from build123d import *

# Parameters (mm, degrees)
CYLINDER904_R               = 1.5
CYLINDER904_DEPTH           = 20
CYLINDER904_PLACEMENT_ANGLE = 45
CYLINDER907_R               = 1.5
CYLINDER907_DEPTH           = 20
CYLINDER902_R               = 1.5
CYLINDER902_DEPTH           = 20
CYLINDER902_PLACEMENT_ANGLE = 135
CYLINDER901_R               = 1.5
CYLINDER901_DEPTH           = 20
CYLINDER903_R               = 1.5
CYLINDER903_DEPTH           = 20
CYLINDER903_PLACEMENT_ANGLE = 225
CYLINDER905_R               = 1.5
CYLINDER905_DEPTH           = 20
CYLINDER906_R               = 1.5
CYLINDER906_DEPTH           = 20
CYLINDER906_PLACEMENT_ANGLE = 45
CYLINDER898_R               = 1.5
CYLINDER898_DEPTH           = 20
COMPOUND256_PLACEMENT_ANGLE = 22.5
BOX408_W                    = 6
BOX408_H                    = 8
BOX408_DEPTH                = 2
BOX408_PLACEMENT_ANGLE      = 45
BOX404_W                    = 6
BOX404_H                    = 8
BOX404_DEPTH                = 2
BOX415_W                    = 6
BOX415_H                    = 8
BOX415_DEPTH                = 2
BOX415_PLACEMENT_ANGLE      = 135
BOX407_W                    = 6
BOX407_H                    = 8
BOX407_DEPTH                = 2
BOX412_W                    = 6
BOX412_H                    = 8
BOX412_DEPTH                = 2
BOX412_PLACEMENT_ANGLE      = 225
BOX128_W                    = 6
BOX128_H                    = 8
BOX128_DEPTH                = 2
BOX414_W                    = 6
BOX414_H                    = 8
BOX414_DEPTH                = 2
BOX414_PLACEMENT_ANGLE      = 45
BOX413_W                    = 6
BOX413_H                    = 8
BOX413_DEPTH                = 2
COMPOUND780_PLACEMENT_ANGLE = 22.5
CYLINDER888_R               = 1.5
CYLINDER888_DEPTH           = 20
CYLINDER897_R               = 1.5
CYLINDER897_DEPTH           = 20
CYLINDER896_R               = 1.5
CYLINDER896_DEPTH           = 20
CYLINDER900_R               = 1.5
CYLINDER900_DEPTH           = 20
BOX409_W                    = 6
BOX409_H                    = 2
BOX409_DEPTH                = 6
BOX406_W                    = 6
BOX406_H                    = 2
BOX406_DEPTH                = 6
BOX411_W                    = 6
BOX411_H                    = 2
BOX411_DEPTH                = 6
BOX410_W                    = 6
BOX410_H                    = 2
BOX410_DEPTH                = 6
TUBE087_R                   = 52
TUBE087_R_2                 = 42
TUBE087_DEPTH               = 8


with BuildPart() as obj1:
    # Cylinder904 → Cylinder904 (new body)
    with BuildSketch(Plane.XY):
        Circle(CYLINDER904_R)
    extrude(amount=CYLINDER904_DEPTH)


with BuildPart() as obj1_1:
    # Cylinder904 placement: moved
    add(obj1.part.moved(Location((-31.819805, 31.819805, -18))).rotate(Axis((-31.819805, 31.819805, -18), (0, 0, 1)), CYLINDER904_PLACEMENT_ANGLE))


with BuildPart() as obj2:
    # Cylinder907 → Cylinder907 (new body)
    with BuildSketch(Plane(origin=(-45, 0, -18), x_dir=(0, 1, 0), z_dir=(0, 0, 1))):
        Circle(CYLINDER907_R)
    extrude(amount=CYLINDER907_DEPTH)


with BuildPart() as obj3:
    # Cylinder902 → Cylinder902 (new body)
    with BuildSketch(Plane.XY):
        Circle(CYLINDER902_R)
    extrude(amount=CYLINDER902_DEPTH)


with BuildPart() as obj3_1:
    # Cylinder902 placement: moved
    add(obj3.part.moved(Location((-31.819805, -31.819805, -18))).rotate(Axis((-31.819805, -31.819805, -18), (0, 0, 1)), CYLINDER902_PLACEMENT_ANGLE))


with BuildPart() as obj4:
    # Cylinder901 → Cylinder901 (new body)
    with BuildSketch(Plane(origin=(0, -45, -18), x_dir=(-1, 0, 0), z_dir=(0, 0, 1))):
        Circle(CYLINDER901_R)
    extrude(amount=CYLINDER901_DEPTH)


with BuildPart() as obj5:
    # Cylinder903 → Cylinder903 (new body)
    with BuildSketch(Plane.XY):
        Circle(CYLINDER903_R)
    extrude(amount=CYLINDER903_DEPTH)


with BuildPart() as obj5_1:
    # Cylinder903 placement: moved
    add(obj5.part.moved(Location((31.819805, -31.819805, -18))).rotate(Axis((31.819805, -31.819805, -18), (0, 0, 1)), CYLINDER903_PLACEMENT_ANGLE))


with BuildPart() as obj6:
    # Cylinder905 → Cylinder905 (new body)
    with BuildSketch(Plane(origin=(45, 0, -18), x_dir=(0, -1, 0), z_dir=(0, 0, 1))):
        Circle(CYLINDER905_R)
    extrude(amount=CYLINDER905_DEPTH)


with BuildPart() as obj7:
    # Cylinder906 → Cylinder906 (new body)
    with BuildSketch(Plane.XY):
        Circle(CYLINDER906_R)
    extrude(amount=CYLINDER906_DEPTH)


with BuildPart() as obj7_1:
    # Cylinder906 placement: moved
    add(obj7.part.moved(Location((31.819805, 31.819805, -18))).rotate(Axis((31.819805, 31.819805, -18), (0, 0, -1)), CYLINDER906_PLACEMENT_ANGLE))


with BuildPart() as compound256:
    # Cylinder898 → Cylinder898 (new body)
    with BuildSketch(Plane(origin=(0, 45, -18), x_dir=(1, 0, 0), z_dir=(0, 0, 1))):
        Circle(CYLINDER898_R)
    extrude(amount=CYLINDER898_DEPTH)

    # Compound256: union obj1, obj2, obj3, obj4, obj5, obj6, obj7
    add(obj1_1.part)
    add(obj2.part)
    add(obj3_1.part)
    add(obj4.part)
    add(obj5_1.part)
    add(obj6.part)
    add(obj7_1.part)


with BuildPart() as compound256_1:
    # Compound256 placement: moved
    add(compound256.part.rotate(Axis((0, 0, 0), (0, 0, 1)), COMPOUND256_PLACEMENT_ANGLE))


with BuildPart() as krychle408:
    # Box408 → Box408 (new body)
    with BuildSketch(Plane.XY):
        with Locations((3, 4)):
            Rectangle(BOX408_W, BOX408_H)
    extrude(amount=BOX408_DEPTH)


with BuildPart() as krychle408_1:
    # Box408 placement: moved
    add(krychle408.part.moved(Location((-31.112698, 26.870058, -4))).rotate(Axis((-31.112698, 26.870058, -4), (0, 0, 1)), BOX408_PLACEMENT_ANGLE))


with BuildPart() as krychle404:
    # Box404 → Box404 (new body)
    with BuildSketch(Plane(origin=(-41, -3, -4), x_dir=(0, 1, 0), z_dir=(0, 0, 1))):
        with Locations((3, 4)):
            Rectangle(BOX404_W, BOX404_H)
    extrude(amount=BOX404_DEPTH)


with BuildPart() as krychle415:
    # Box415 → Box415 (new body)
    with BuildSketch(Plane.XY):
        with Locations((3, 4)):
            Rectangle(BOX415_W, BOX415_H)
    extrude(amount=BOX415_DEPTH)


with BuildPart() as krychle415_1:
    # Box415 placement: moved
    add(krychle415.part.moved(Location((-26.870058, -31.112698, -4))).rotate(Axis((-26.870058, -31.112698, -4), (0, 0, 1)), BOX415_PLACEMENT_ANGLE))


with BuildPart() as krychle407:
    # Box407 → Box407 (new body)
    with BuildSketch(Plane(origin=(3, -41, -4), x_dir=(-1, 0, 0), z_dir=(0, 0, 1))):
        with Locations((3, 4)):
            Rectangle(BOX407_W, BOX407_H)
    extrude(amount=BOX407_DEPTH)


with BuildPart() as krychle412:
    # Box412 → Box412 (new body)
    with BuildSketch(Plane.XY):
        with Locations((3, 4)):
            Rectangle(BOX412_W, BOX412_H)
    extrude(amount=BOX412_DEPTH)


with BuildPart() as krychle412_1:
    # Box412 placement: moved
    add(krychle412.part.moved(Location((31.112698, -26.870058, -4))).rotate(Axis((31.112698, -26.870058, -4), (0, 0, 1)), BOX412_PLACEMENT_ANGLE))


with BuildPart() as krychle128:
    # Box128 → Box128 (new body)
    with BuildSketch(Plane(origin=(41, 3, -4), x_dir=(0, -1, 0), z_dir=(0, 0, 1))):
        with Locations((3, 4)):
            Rectangle(BOX128_W, BOX128_H)
    extrude(amount=BOX128_DEPTH)


with BuildPart() as krychle414:
    # Box414 → Box414 (new body)
    with BuildSketch(Plane.XY):
        with Locations((3, 4)):
            Rectangle(BOX414_W, BOX414_H)
    extrude(amount=BOX414_DEPTH)


with BuildPart() as krychle414_1:
    # Box414 placement: moved
    add(krychle414.part.moved(Location((26.870058, 31.112698, -4))).rotate(Axis((26.870058, 31.112698, -4), (0, 0, -1)), BOX414_PLACEMENT_ANGLE))


with BuildPart() as compound780:
    # Box413 → Box413 (new body)
    with BuildSketch(Plane(origin=(-3, 41, -4), x_dir=(1, 0, 0), z_dir=(0, 0, 1))):
        with Locations((3, 4)):
            Rectangle(BOX413_W, BOX413_H)
    extrude(amount=BOX413_DEPTH)

    # Compound780: union Krychle408, Krychle404, Krychle415, Krychle407, Krychle412, Krychle128, Krychle414
    add(krychle408_1.part)
    add(krychle404.part)
    add(krychle415_1.part)
    add(krychle407.part)
    add(krychle412_1.part)
    add(krychle128.part)
    add(krychle414_1.part)


with BuildPart() as compound780_1:
    # Compound780 placement: moved
    add(compound780.part.rotate(Axis((0, 0, 0), (0, 0, 1)), COMPOUND780_PLACEMENT_ANGLE))


with BuildPart() as obj8:
    # Cylinder888 → Cylinder888 (new body)
    with BuildSketch(Plane(origin=(24, -40, -5), x_dir=(1, 0, 0), z_dir=(0, -1, 0))):
        Circle(CYLINDER888_R)
    extrude(amount=CYLINDER888_DEPTH)


with BuildPart() as obj9:
    # Cylinder897 → Cylinder897 (new body)
    with BuildSketch(Plane(origin=(51, -40, 7), x_dir=(1, 0, 0), z_dir=(0, -1, 0))):
        Circle(CYLINDER897_R)
    extrude(amount=CYLINDER897_DEPTH)


with BuildPart() as obj10:
    # Cylinder896 → Cylinder896 (new body)
    with BuildSketch(Plane(origin=(-51, -40, 7), x_dir=(1, 0, 0), z_dir=(0, -1, 0))):
        Circle(CYLINDER896_R)
    extrude(amount=CYLINDER896_DEPTH)


with BuildPart() as compound255:
    # Cylinder900 → Cylinder900 (new body)
    with BuildSketch(Plane(origin=(-24, -40, -5), x_dir=(1, 0, 0), z_dir=(0, -1, 0))):
        Circle(CYLINDER900_R)
    extrude(amount=CYLINDER900_DEPTH)

    # Compound255: union obj8, obj9, obj10
    add(obj8.part)
    add(obj9.part)
    add(obj10.part)


with BuildPart() as krychle409:
    # Box409 → Box409 (new body)
    with BuildSketch(Plane(origin=(21, -47, -8), x_dir=(1, 0, 0), z_dir=(0, 0, 1))):
        with Locations((3, 1)):
            Rectangle(BOX409_W, BOX409_H)
    extrude(amount=BOX409_DEPTH)


with BuildPart() as krychle406:
    # Box406 → Box406 (new body)
    with BuildSketch(Plane(origin=(48, -45, 4), x_dir=(1, 0, 0), z_dir=(0, 0, 1))):
        with Locations((3, 1)):
            Rectangle(BOX406_W, BOX406_H)
    extrude(amount=BOX406_DEPTH)


with BuildPart() as krychle411:
    # Box411 → Box411 (new body)
    with BuildSketch(Plane(origin=(-54, -45, 4), x_dir=(1, 0, 0), z_dir=(0, 0, 1))):
        with Locations((3, 1)):
            Rectangle(BOX411_W, BOX411_H)
    extrude(amount=BOX411_DEPTH)


with BuildPart() as compound257:
    # Box410 → Box410 (new body)
    with BuildSketch(Plane(origin=(-27, -47, -8), x_dir=(1, 0, 0), z_dir=(0, 0, 1))):
        with Locations((3, 1)):
            Rectangle(BOX410_W, BOX410_H)
    extrude(amount=BOX410_DEPTH)

    # Compound257: union Krychle409, Krychle406, Krychle411
    add(krychle409.part)
    add(krychle406.part)
    add(krychle411.part)


with BuildPart() as cut145:
    # Tube087 → Tube087 (new body)
    with BuildSketch(Plane.XY.offset(-8)):
        Circle(TUBE087_R)
        Circle(TUBE087_R_2, mode=Mode.SUBTRACT)
    extrude(amount=TUBE087_DEPTH)

    # Cut407: cut Compound257
    add(compound257.part, mode=Mode.SUBTRACT)

    # Cut144: cut Compound255
    add(compound255.part, mode=Mode.SUBTRACT)

    # Cut404: cut Compound780
    add(compound780_1.part, mode=Mode.SUBTRACT)

    # Cut145: cut Compound256
    add(compound256_1.part, mode=Mode.SUBTRACT)


solid = cut145.part
Can you work these out from the model? Positions are in its coordinate system, mm. A direction names the side the tool comes from. Round coordinates to 2 decimals unless told otherwise and drop trailing zeros. Order: outer loops, then holes, each group sorted by start corner. A loop starts at its lowest first (then second) coordinate and runs counter-clockwise, first axis right, second up. Notation, with made-up numbers: (49, 24.5) -> (60, 24.5) arc R13 cw to (60, 37.5) -> close; hole circle Ø2 at (62, -27.5). An arc over 180 degrees is marked (long way). Write each question's results on one line, items separated by ' | '. Start each with the question number.
Item 1: Will these pins go through, and if not, where does the flat tip stop? pin 1 (3.5 mm diameter, centred on x = -24, z = -5, fed in from +Y); pin 2 (3 mm diameter, centred on x = -35, z = -1.5, fed in from -Y); pin 3 (1.5 mm diameter, centred on y = 15, z = -4, fed in from +X); pin 4 (1 mm diameter, centred on x = 36, y = -17, fed in from -Z).
Item 2: If we section it at C-C, the plane x = -24: Write out the boundary of the cut face in (y, z).
Item 3: Which directions (+Z, -Z, +X, -X, +Y, -Y) give clear straight access to the entire face, cutting with the end or side of a thin tool? Please do faces 1 (the cylindrical face through (-17.609, -43.023, -1.014)), 2 (the flat face through (-45.254, -18.79, -3.014)).
Item 4: Thinking about a two-plate mould opening in Z: for faces 3 (the flat face through (18.79, -45.254, -3.014)), 4 (the cylindrical face through (-40.097, -16.961, -1.014)), which applies, +Z half, -Z half, draft (parallel to the pull), parting line (faces both ways), or undercut?
Item 5: Please list where these lines run through material, in increasing order: L1, parallel to Z at x = 24, y = -41.45; L2, parallel to Y at x = -31, z = -1.75; L3, parallel to X at y = -46.5, z = -3.75.
Item 6: If we section it at A-A, the plane x = 0: Write out the boundary of the cut face in (y, z).
Results:
1) pin 1: stops at y = 47 | pin 2: stops at y = -39.77 | pin 3: stops at x = 50.01 | pin 4: passes through
2) outline: (-46.13, -2) -> (-45, -2) -> (-45, -3.5) -> (-40, -3.5) -> (-40, -6.5) -> (-45, -6.5) -> (-45, -8) -> (-34.47, -8) -> (-34.47, 0) -> (-46.13, 0) -> close; (34.47, -8) -> (46.13, -8) -> (46.13, 0) -> (34.47, 0) -> close
3) face 1: +Z, -Z | face 2: none
4) face 3: undercut | face 4: draft
5) L1: z = -8 to -6.5, -3.5 to 0 | L2: y = -41.75 to -28.34, 28.34 to 41.75 | L3: x = -21 to 21
6) outline: (-52, -8) -> (-42, -8) -> (-42, 0) -> (-52, 0) -> close; (42, -8) -> (52, -8) -> (52, 0) -> (42, 0) -> close
